from build123d import *

# Parameters (mm, degrees)
BOSS_EXTRUDE1_DEPTH = 19.812
SKETCH2_R           = 2.921
BOSS_EXTRUDE2_DEPTH = 9.906


with BuildPart() as part:
    # Sketch1 → Boss-Extrude1 (new body)
    with BuildSketch(Plane(origin=(0, 0, 0), x_dir=(1, 0, 0), z_dir=(0, 1, 0))):
        with BuildLine():
            ThreePointArc((-38.1, -35.603754118), (-12.026846627, -25.317436869), (0, 0))
            Line((0, 0), (-38.1, 0))
            Line((-38.1, 0), (-38.1, -6.604))
            ThreePointArc((-38.1, -6.604), (-31.095400226, -9.505400226), (-28.194, -16.51))
            ThreePointArc((-28.194, -16.51), (-31.095400226, -23.514599774), (-38.1, -26.416))
            Line((-38.1, -26.416), (-38.1, -35.603754118))
        make_face()
        with BuildLine():
            Line((-38.1, -6.604), (-38.1, 0))
            Line((-38.1, 0), (-76.2, 0))
            ThreePointArc((-76.2, 0), (-64.173153373, -25.317436869), (-38.1, -35.603754118))
            Line((-38.1, -35.603754118), (-38.1, -26.416))
            ThreePointArc((-38.1, -26.416), (-48.006, -16.51), (-38.1, -6.604))
        make_face()
    extrude(amount=BOSS_EXTRUDE1_DEPTH)

    # Sketch2 → Boss-Extrude2 (add)
    with BuildSketch(Plane(origin=(0, 0, 0), x_dir=(-1, 0, 0), z_dir=(0, 0, -1))):
        Polygon((0, 0), (0, -69.85), (76.2, -69.85), (76.2, 0), (76.2, 31.75), (0, 31.75), align=None)
        with Locations((9.906, -44.45)):
            Circle(SKETCH2_R, mode=Mode.SUBTRACT)
        with Locations((66.294, -44.45)):
            Circle(SKETCH2_R, mode=Mode.SUBTRACT)
    extrude(amount=BOSS_EXTRUDE2_DEPTH)


solid = part.part
Here's how the part is built. I have some questions about the finished solid (model axes, mm). A direction names the side the tool comes from. Give positions to 0.01 mm unless a question says otherwise; leave off trailing zeros. Loops run counter-clockwise (first coordinate to the right, second up) from the corner with the lowest first, then second, coordinate; pieces in that order, holes last. Notation, with made-up numbers: (63, -16) -> (100, -16) arc R28 ccw to (100, 8) -> close; hole circle Ø1 at (-19.5, 1). An arc over 180 degrees is marked (long way). Answer as a JSON object with one key per item and string values. Group by question number.
Item 1: Imagine slicing it at C-C on x = -25. Write out the boundary of the cut face in (y, z), then the cut area to 3 significant figures.
Item 2: Imagine slicing it at B-B on y = 15.5. Write out the boundary of the cut face in (x, z).
Item 3: I need wall thicknesses on L1, parallel to Y at x = -46, z = 23; L2, parallel to Z at x = -52, y = -64; L3, parallel to X at y = -44, z = -3. Which ranges of each line are inside material? Lowest first, please.
Item 4: Thinking about a two-plate mould opening in Y: for faces 3 (the cylindrical face through (-11.254, -47.041, -4.884)), 4 (the cylindrical face through (-68.99, -45.57, -4.88)), 5 (the flat face through (-38, 26, 0)), 6 (the flat face through (-39, 19.812, 6)), which applies, pulls with the +Y half, pulls with the -Y half, needs draft (parallel to the pull), parting line crosses it, or undercut?
Item 5: Will these pins go through, and if not, where does the flat tip stop? pin 1 (1 mm diameter, centred on x = -30.5, z = 20.5, fed in from -Y); pin 2 (6.5 mm diameter, centred on x = -9.906, y = -44.45, fed in from -Z); pin 3 (5 mm diameter, centred on x = -62.5, y = 12.5, fed in from +Z); pin 4 (6 mm diameter, centred on x = -58.5, z = 26, fed in from -Y).
Item 6: Imagine slicing it at D-D on z = 1.5. Write out the boundary of the cut face in (x, y), then the cut area to 3 significant figures.
Item 7: On a 3-axis mill with a long thin cutter (end or side, diameter ignored), from which of +Z, -Z, +X, -X, +Y, -Y can I reach the whole of each face in a straight line? I mean faces 1 (the flat face through (-39, 0, 6)), 2 (the flat face through (-76.2, -20, -5)). Say none if no direction works.
Item 8: Imagine slicing it at A-A on y = -44.45. Write out the boundary of the cut face in (x, z) (3 decimals), then the cut area to 3 significant figures.
Answer list:
{
 "1": {"outline": "(-69.85, -9.91) -> (31.75, -9.91) -> (31.75, 0) -> (19.81, 0) -> (19.81, 33.29) -> (0, 33.29) -> (0, 0) -> (-69.85, 0) -> close", "area": "1,670 mm2"},
 "2": {"outline": "(-76.2, -9.91) -> (0, -9.91) -> (0, 0) arc R38.19 ccw to (-76.2, 0) -> close; hole circle Ø19.81 at (-38.1, 16.51)"},
 "3": {"L1": "y = 0 to 19.81", "L2": "z = -9.91 to 0", "L3": "x = -76.2 to -69.18, -63.41 to -12.79, -7.02 to 0"},
 "4": {"face 3": "undercut", "face 4": "undercut", "face 5": "needs draft", "face 6": "pulls with the +Y half"},
 "5": {"pin 1": "passes through", "pin 2": "stops at z = -9.91", "pin 3": "stops at z = 28.7", "pin 4": "stops at y = 0"},
 "6": {"outline": "(-76.07, 0) -> (-0.13, 0) -> (-0.13, 19.81) -> (-76.07, 19.81) -> close", "area": "1,500 mm2"},
 "7": {"face 1": "+Z, +X, -X, -Y", "face 2": "+Z, -Z, -X, +Y, -Y"},
 "8": {"outline": "(-76.2, -9.906) -> (-69.215, -9.906) -> (-69.215, 0) -> (-76.2, 0) -> close; (-63.373, -9.906) -> (-12.827, -9.906) -> (-12.827, 0) -> (-63.373, 0) -> close; (-6.985, -9.906) -> (0, -9.906) -> (0, 0) -> (-6.985, 0) -> close", "area": "639 mm2"}
}
